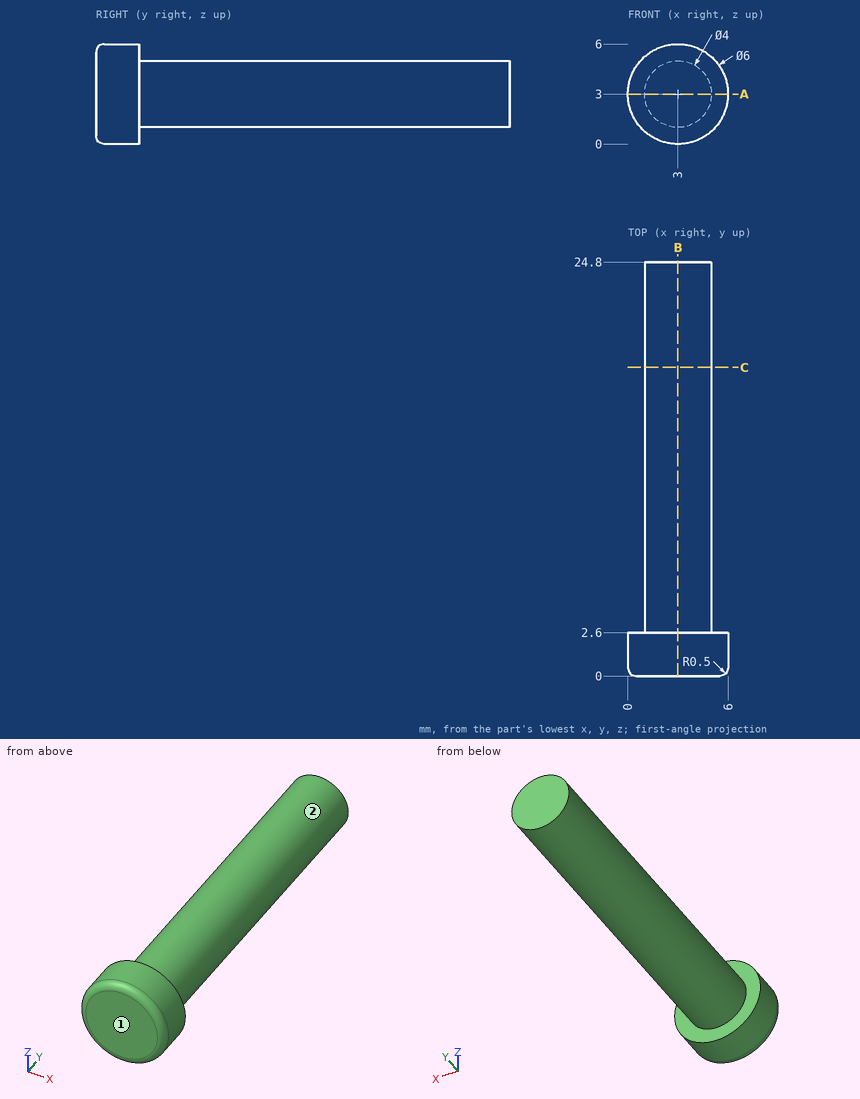
Can you work these out from the drawing? Everything is in mm from the part's minimum corner. A direction names the side the tool comes from. Coordinates: 2 decimals unless noted, no trailing zeros. Write each loop counter-clockwise with the first axis right and the second up, starting at its lowest first coordinate (ties: lowest second). Pieces come first, ordered by that corner, then holes. Notation, with made-up numbers: (-6, 57) -> (53, 57) arc R16 cw to (53, 78) -> close; hole circle Ø3 at (-6, 13). An arc over 180 degrees is marked (long way). Write item = value, one per line.
(1) If I drill on probe 1 along X at (y, z) = (21.75, 3.15); probe 2 along X at (y, z) = (7, 4.2); probe 3 along Y at (x, z) = (4.15, 4.8), over which ranges is the centre line in solid material (lowest first)?
Verdict:
probe_1 = 1.01 to 4.99
probe_2 = 1.4 to 4.6
probe_3 = 0 to 2.6
(2) Imagine slicing it at A-A (z = 3). Please give me the cut outline in (x, y).
Verdict:
outline = (0, 0.5) arc R0.5 ccw to (0.5, 0) -> (5.5, 0) arc R0.5 ccw to (6, 0.5) -> (6, 2.6) -> (5, 2.6) -> (5, 24.8) -> (1, 24.8) -> (1, 2.6) -> (0, 2.6) -> close
(3) Imagine slicing it at C-C (y = 18.5). Please give me the cut outline in (x, z).
Verdict:
outline = circle Ø4 at (3, 3)
(4) On a 3-axis mill with a long thin cutter (end or side, diameter ignored), from which of +Z, -Z, +X, -X, +Y, -Y can I reach the whole of each face in a straight line? I mean the marked faces 1 and 2. Say none if no direction works.
Verdict:
face_1 = +Z, -Z, +X, -X, -Y
face_2 = +Y
(5) For pin 1 (1 mm diameter, centred on y = 7, z = 4, fed in from +X); pin 2 (2 mm diameter, centred on x = 5, y = 17.5, fed in from +Z); pin 3 (3 mm diameter, centred on y = 10.5, z = 1, fed in from -X), each with a flat end and sliding along its axis, tell me the tip position at first contact or that it passes through.
Verdict:
pin_1 = 4.94
pin_2 = 4.73
pin_3 = 1.06
(6) Imagine slicing it at B-B (x = 3). Please give me the cut outline in (y, z).
Verdict:
outline = (0, 0.5) arc R0.5 ccw to (0.5, 0) -> (2.6, 0) -> (2.6, 1) -> (24.8, 1) -> (24.8, 5) -> (2.6, 5) -> (2.6, 6) -> (0.5, 6) arc R0.5 ccw to (0, 5.5) -> close
